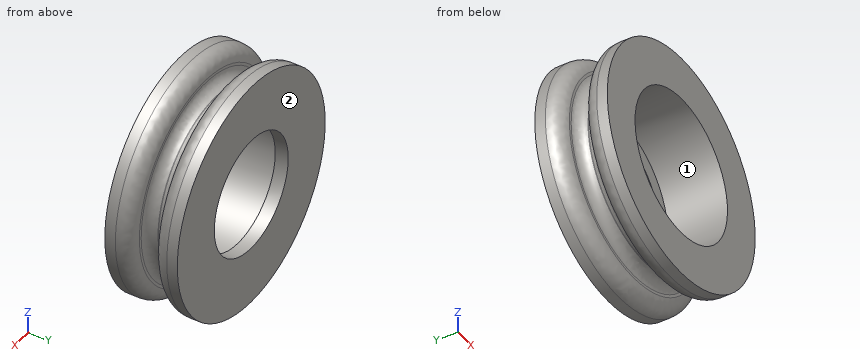
from build123d import *

# Parameters (mm, degrees)
FILLET5_R = 2.286
FILLET6_R = 1.6002


with BuildPart() as part:
    # Sketch2 → Revolve1 (revolve)
    with BuildSketch(Plane(origin=(0, 0, 0), x_dir=(0, 0, -1), z_dir=(1, 0, 0))):
        Polygon((8.89, 5.55752), (8.89, 3.5687), (11.1125, 3.5687), (11.1125, -5.55752), (17.78, -5.55752), (17.78, -1.7399), (13.639699492, -1.57734), (13.639699492, 1.57734), (17.78, 1.7399), (17.78, 5.55752), align=None)
    revolve(axis=Axis((0, 16.043148, 0), (0, -1, 0)))

    # Fillet5
    fillet5_edges = [part.edges().sort_by_distance(p)[0] for p in [
        (0, 1.7399, 17.78),
        (0, -1.7399, 17.78),
    ]]
    fillet(fillet5_edges, radius=FILLET5_R)

    # Fillet6
    fillet6_edges = [part.edges().sort_by_distance(p)[0] for p in [
        (0, 1.57734, 13.639699492),
        (0, -1.57734, 13.639699492),
    ]]
    fillet(fillet6_edges, radius=FILLET6_R)


solid = part.part
The listing builds one solid part. Answer for the finished solid, in the listing's coordinates (mm). Face numbers are marked on the shaded views. Give positions to 0.01 mm unless a question says otherwise; leave off trailing zeros. Write each loop counter-clockwise with the first axis right and the second up, starting at its lowest first coordinate (ties: lowest second). Pieces come first, ordered by that corner, then holes. Notation, with made-up numbers: (29.25, 7) - (80.25, 7) arc R10 cw to (80.25, 19) - close; hole circle Ø8 at (81.25, -26.75). An arc over 180 degrees is marked (long way). Use a Markdown table: item, result.
1. For a pull along Z with two mould halves and no side action, classify the marked faces 1 and 2 as released by +Z, released by -Z, zero draft, split by the parting line, or undercut.
Values follow:
| item | result |
|---|---|
| face 1 | undercut |
| face 2 | zero draft |
2. Find the intervals of material crossed by probe 1 along Y at (x, z) = (10.5, 11); probe 2 along Z at (x, y) = (3.5, 2); probe 3 along Y at (x, z) = (8.5, -7), in increasing order. Write a range as from..to.
Values follow:
| item | result |
|---|---|
| probe 1 | y = -5.56..-1.64, 1.64..5.56 |
| probe 2 | z = -16.34..-10.55, 10.55..16.34 |
| probe 3 | y = 3.57..5.56 |
3. Each of these flat-tipped pins is pushed along its axis until it touches: P1, Ø14, axis at x = 0, z = 0, coming from the -Y side; P2, Ø3, axis at x = 1, y = 0.5, coming from the -Z side; P3, Ø20, axis at x = 0, z = 0, coming from the -Y side; P4, Ø3, axis at x = 3, y = -4.5, coming from the +Z side. Where does it stop, or does it pass through?
Values follow:
| item | result |
|---|---|
| P1 | passes through |
| P2 | stops at z = -16.68 |
| P3 | stops at y = 3.57 |
| P4 | stops at z = 17.72 |
4. Section A-A on y = 4.75 is taken. Write down the section's boundary in (x, z).
Values follow:
| item | result |
|---|---|
| outline | circle Ø35.56 at (0, 0); hole circle Ø17.78 at (0, 0) |
